Work out the finished part from the listing and answer in its coordinate system (mm). A direction names the side the tool comes from. Give positions to 0.01 mm unless a question says otherwise; leave off trailing zeros. Loops run counter-clockwise (first coordinate to the right, second up) from the corner with the lowest first, then second, coordinate; pieces in that order, holes last. Notation, with made-up numbers: (-4, -1) - (5, -1) arc R26 cw to (5, 34) - close; hole circle Ø3 at (85, 40). An arc over 180 degrees is marked (long way). One line per question, with ' | ' between items. Start each with the question number.
1. Each of these flat-tipped pins is pushed along its axis until it touches: pin 1 (6.5 mm diameter, centred on x = -2, y = 5.5, fed in from -Z); pin 2 (10 mm diameter, centred on x = -12.5, z = -32.5, fed in from -Y); pin 3 (9 mm diameter, centred on y = -0.5, z = -56, fed in from +X). Where does it stop, or does it pass through?
2. Section D-D (z = -52.5) is taken. Determine the outline of the cut face in (x, y).
3. Section C-C (y = -7) is taken. Determine the outline of the cut face in (x, z).
4. Section B-B (y = 5.25) is taken. Determine the outline of the cut face in (x, z), plus the area to 3 significant figures.
5. Which of the six approach directions +Z, -Z, +X, -X, +Y, -Y give full straight-line access (tool end or side, diameter ignored) to faces 4 (the face through (-6, -8, -55)), 5 (the face through (-2, 6, -9.7)), 6 (the face through (2.38, -10.74, -30.21)), 7 (the face through (0, 0, 0)), 8 (the face through (-6, 8, -55))?
6. Section A-A (x = -9.25) is taken. Determine the outline of the cut face in (y, z).
7. Find the intervals of material crossed by line 1 (Z direction, x = 1.75, y = -7); line 2 (Z direction, x = -4, y = -7); line 3 (Z direction, x = -3, y = 1.75), in increasing order.
8. For a pull along Z with two mould halves and no side action, classify faces 1 (the face through (-0.18, 0.79, -63.49)), 2 (the face through (4.5, 0, -55)), 3 (the face through (0.59, 4.46, -13.97)) as released by +Z, released by -Z, zero draft, split by the parting line, or undercut.
from build123d import *

# Parameters (mm, degrees)
F2_W     = 20
F2_H     = 16
F3_DEPTH = 11.5
F4_R     = 3


# Not quite as in the source:
# - an extrude whose draft closes it to a point is written as a loft to that point


with BuildPart() as f1:
    # F0 (on Front) → F1 (revolve)
    with BuildSketch(Plane.XZ):
        Polygon((0, -49.8), (0, 0), (-8, 0), (-8, -3.7), (-6, -3.7), (-6, -9.7), (-8, -9.7), (-8, -12.7), (-4.5, -12.7), (-4.5, -15.2), (-11, -15.2), (-11, -44.8), (-3, -44.8), (-3, -49.8), align=None)
    revolve(axis=Axis((0, 0, -24.9), (0, 0, -1)))

    # F2 (on face) → F3 (join)
    with BuildSketch(Plane(origin=(0, 0, -49.8), x_dir=(1, 0, 0), z_dir=(0, 0, -1))):
        with Locations((-5.5, 0)):
            Rectangle(F2_W, F2_H)
    extrude(amount=F3_DEPTH)

    # F4 (on face) → F5 section 0
    with BuildSketch(Plane(origin=(0, 0, -61.3), x_dir=(1, 0, 0), z_dir=(0, 0, -1)), mode=Mode.PRIVATE) as f5_s0:
        Circle(F4_R)
    loft([f5_s0.sketch, Vertex(0, 0, -64.3)], ruled=True)


solid = f1.part
Conclusion:
1) pin 1: z = -61.7 | pin 2: y = -8.05 | pin 3: x = 4.5
2) outline: (-15.5, -8) - (4.5, -8) - (4.5, 8) - (-15.5, 8) - close
3) outline: (-15.5, -61.3) - (4.5, -61.3) - (4.5, -49.8) - (-15.5, -49.8) - close; (-8.49, -44.8) - (8.49, -44.8) - (8.49, -15.2) - (-8.49, -15.2) - close; (-3.87, -12.7) - (3.87, -12.7) - (3.87, -9.7) - (-3.87, -9.7) - close; (-3.87, -3.7) - (3.87, -3.7) - (3.87, 0) - (-3.87, 0) - close
4) outline: (-15.5, -61.3) - (4.5, -61.3) - (4.5, -49.8) - (-15.5, -49.8) - close; (-9.67, -44.8) - (9.67, -44.8) - (9.67, -15.2) - (-9.67, -15.2) - close; (-6.04, -12.7) - (6.04, -12.7) - (6.04, -9.7) - (2.9, -9.7) - (2.9, -3.7) - (6.04, -3.7) - (6.04, 0) - (-6.04, 0) - (-6.04, -3.7) - (-2.9, -3.7) - (-2.9, -9.7) - (-6.04, -9.7) - close | area: 918 mm²
5) face 4: -Z, +X, -X, -Y | face 5: none | face 6: +Z | face 7: +Z, +X, -X, +Y, -Y | face 8: -Z, +X, -X, +Y
6) outline: (-8, -61.3) - (8, -61.3) - (8, -49.8) - (-8, -49.8) - close; (-5.95, -44.8) - (5.95, -44.8) - (5.95, -15.2) - (-5.95, -15.2) - close
7) line 1: -61.3 to -49.8, -44.8 to -15.2, -12.7 to -9.7, -3.7 to 0 | line 2: -61.3 to -49.8, -44.8 to -15.2 | line 3: -61.3 to -49.8, -44.8 to 0
8) face 1: released by -Z | face 2: zero draft | face 3: undercut
